Geometry check sheet. Reference: drawing and pictorial views, mm from the part's lowest x, y, z. Give positions to 0.01 mm unless a question says otherwise; leave off trailing zeros. Order: outer loops, then holes, each group sorted by start corner. A loop starts at its lowest first (then second) coordinate and runs counter-clockwise, first axis right, second up. Notation, with made-up numbers: (34.5, 64.25) - (71.5, 64.25) arc R24 ccw to (71.5, 78.25) - close; hole circle Ø3 at (-18, -19.5). An arc over 180 degrees is marked (long way). Answer as a JSON object with one key per item and string values.
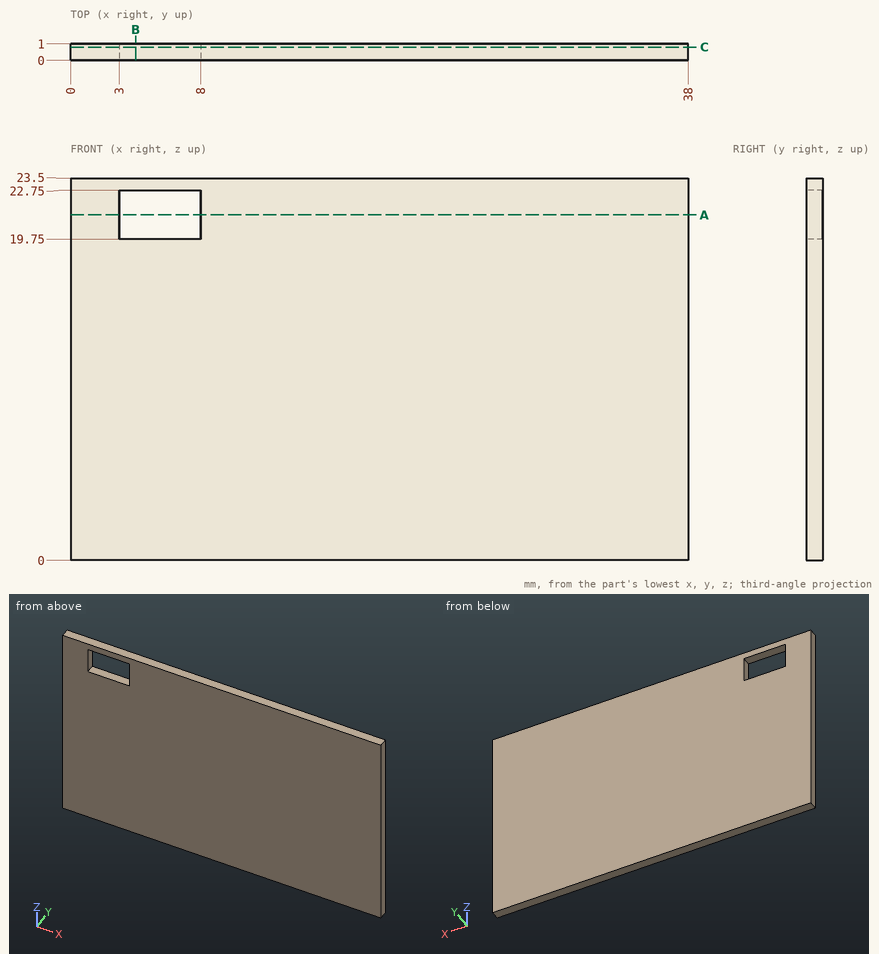
(1) Section check C-C (y = 0.8). Record the cut outline in (x, z).
Computed values:
{"outline": "(0, 0) - (38, 0) - (38, 23.5) - (0, 23.5) - close; hole (3, 19.75) - (8, 19.75) - (8, 22.75) - (3, 22.75) - close"}
(2) Section check A-A (z = 21.25). Record the cut outline in (x, y).
Computed values:
{"outline": "(0, 0) - (3, 0) - (3, 1) - (0, 1) - close; (8, 0) - (38, 0) - (38, 1) - (8, 1) - close"}
(3) Section check B-B (x = 4). Record the cut outline in (y, z), then the cut area to 3 significant figures.
Computed values:
{"outline": "(0, 0) - (1, 0) - (1, 19.75) - (0, 19.75) - close; (0, 22.75) - (1, 22.75) - (1, 23.5) - (0, 23.5) - close", "area": "20.5 mm²"}
(4) Material ranges on line 1 along Z through (x, y) = (7, 0.85); line 2 along X through (y, z) = (0.65, 21.5), recorded low to high. Write a range as [from, to].
Computed values:
{"line 1": "z = [0, 19.75], [22.75, 23.5]", "line 2": "x = [0, 3], [8, 38]"}
